Geometry check sheet. Reference: the model listing, model coordinates, mm. A direction names the side the tool comes from. Round coordinates to 2 decimals unless told otherwise and drop trailing zeros. Order: outer loops, then holes, each group sorted by start corner. A loop starts at its lowest first (then second) coordinate and runs counter-clockwise, first axis right, second up. Notation, with made-up numbers: M 43.25,40.5 L 90.25,40.5 A13 cw 90.25,57.5 Z; hole C 84,-33 d4. An arc over 180 degrees is marked long. Answer as a JSON object with one key per item and string values. Group by question number.
```python
from build123d import *

# Parameters (mm, degrees)
F1_DEPTH = 8
F3_W     = 8
F3_H     = 8
F3_R     = 2.4
F4_DEPTH = 1.7
F5_R     = 2.4
F6_DEPTH = 1.7


with BuildPart() as f1:
    # F0 (on Front) → F1 (new body)
    with BuildSketch(Plane.XZ):
        Polygon((-2.4, 9.6), (-4, 9.6), (-4, 0), (4, 0), (4, 9.6), (2.4, 9.6), (2.4, 11.3), (-2.4, 11.3), align=None)
    extrude(amount=F1_DEPTH)

    # F3 (on plane+point) → F4 (cut, through all)
    with BuildSketch(Plane.XY.offset(11.3)):
        with Locations((0, -4)):
            Rectangle(F3_W, F3_H)
        with Locations((0, -4)):
            Circle(F3_R, mode=Mode.SUBTRACT)
    extrude(amount=-F4_DEPTH, mode=Mode.SUBTRACT)

    # F5 (on Top) → F6 (cut)
    with BuildSketch(Plane.XY):
        with Locations((0, -4)):
            Circle(F5_R)
    extrude(amount=F6_DEPTH, mode=Mode.SUBTRACT)

    # F8: F1 across plane


with BuildPart() as f1_1:
    add(f1.part)
    add(f1.part.mirror(Plane.YZ.offset(4)))


solid = f1_1.part
```
1) Sectioned sample at B-B (y = -5). Record the boundary of the cut face in (x, z).
2) Go/stop test with flat-tipped pins: P1, Ø4, axis at x = 9, y = -5, coming from the -Z side; P2, Ø1.5, axis at x = 3.5, y = -3, coming from the +Z side. Record where each tip stops, or that it passes through.
3) Sectioned sample at A-A (x = 8). Record the boundary of the cut face in (y, z).
4) Release check for a two-part mould opening along X. For faces 1 (the cylindrical face through (10.398, -3.894, 0.838)), 2 (the flat face through (4, -4, 0)), 3 (the flat face through (12, -4, 5)) record: +X half, -X half, draft (parallel to the pull), parting line (faces both ways), or undercut.
5) Set-up check for faces 4 (the cylindrical face through (1.29, -1.976, 0.838)), 5 (the flat face through (-4, -4, 5)), 6 (the flat face through (4, -4, 9.6)): record each of +Z, -Z, +X, -X, +Y, -Y from which the full face is reachable in a straight line by a thin tool's end or side.
6) Thickness scan on line 1 along X through (y, z) = (-6, 1.5); line 2 along Z through (x, y) = (9, -4.25); line 3 along Z through (x, y) = (2.5, -1.5). Record the ranges inside material, lowest first. Write a range as [from, to].
Final values:
{
 "1": {"outline": "M -4,0 L -2.18,0 L -2.18,1.7 L 2.18,1.7 L 2.18,0 L 5.82,0 L 5.82,1.7 L 10.18,1.7 L 10.18,0 L 12,0 L 12,9.6 L 10.18,9.6 L 10.18,11.3 L 5.82,11.3 L 5.82,9.6 L 2.18,9.6 L 2.18,11.3 L -2.18,11.3 L -2.18,9.6 L -4,9.6 Z"},
 "2": {"P1": "stops at z = 0", "P2": "stops at z = 9.6"},
 "3": {"outline": "M -8,0 L -6.4,0 L -6.4,1.7 L -1.6,1.7 L -1.6,0 L 0,0 L 0,9.6 L -1.6,9.6 L -1.6,11.3 L -6.4,11.3 L -6.4,9.6 L -8,9.6 Z"},
 "4": {"face 1": "undercut", "face 2": "draft", "face 3": "+X half"},
 "5": {"face 4": "-Z", "face 5": "+Z, -Z, -X, +Y, -Y", "face 6": "+Z"},
 "6": {"line 1": "x = [-4, -1.33], [1.33, 6.67], [9.33, 12]", "line 2": "z = [1.7, 11.3]", "line 3": "z = [0, 9.6]"}
}
